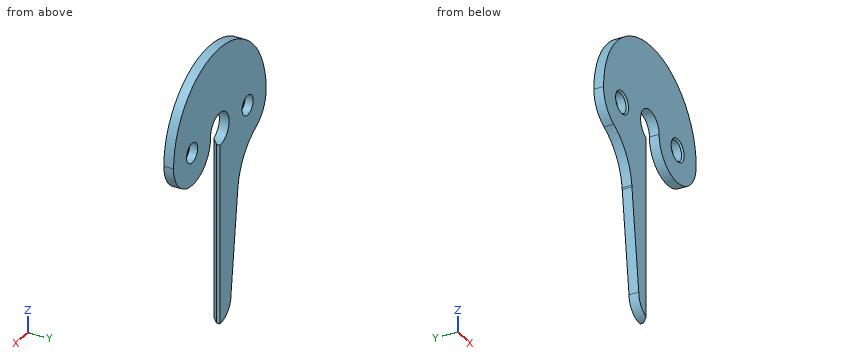
```python
from build123d import *

# Parameters (mm, degrees)
F0_R     = 3
F1_DEPTH = 3
F2_SIZE  = 2
F3_SIZE  = 0.5


with BuildPart() as f1:
    # F0 (on Front) → F1 (new body)
    with BuildSketch(Plane.XZ):
        with BuildLine():
            ThreePointArc((0, -5), (-3.535534, 3.535534), (5, 0))
            ThreePointArc((5, 0), (15, -10), (25, 0))
            ThreePointArc((25, 0), (0, 25), (-25, 0))
            ThreePointArc((-25, 0), (-23.515691, -5.242423), (-19.5034, -8.928571))
            ThreePointArc((-19.5034, -8.928571), (-12.871812, -14.665594), (-9.737763, -22.855169))
            Line((-9.737763, -22.855169), (-9.676577, -23.364999))
            Line((-9.676577, -23.364999), (-6, -54))
            ThreePointArc((-6, -54), (-4.242641, -58.242641), (0, -60))
            Line((0, -60), (0, -5))
        make_face()
        with Locations((-15, 0)):
            Circle(F0_R, mode=Mode.SUBTRACT)
        with Locations((15, 0)):
            Circle(F0_R, mode=Mode.SUBTRACT)
    extrude(amount=F1_DEPTH)

    # F2
    f2_edges = [f1.edges().sort_by_distance(p)[0] for p in [
        (0, -3, -32.5),
    ]]
    chamfer(f2_edges, length=F2_SIZE)

    # F3
    f3_edges = [f1.edges().sort_by_distance(p)[0] for p in [
        (-18, -3, 0),
        (12, -3, 0),
    ]]
    chamfer(f3_edges, length=F3_SIZE)


solid = f1.part
```
Check sheet for the modelled part. Datum: model origin and axes. Units: mm. Round coordinates to 2 decimals unless told otherwise and drop trailing zeros. Order: outer loops, then holes, each group sorted by start corner. A loop starts at its lowest first (then second) coordinate and runs counter-clockwise, first axis right, second up. Notation, with made-up numbers: (13.5, 61.5) - (62.5, 61.5) arc R30 ccw to (62.5, 90.5) - close; hole circle Ø8 at (47, 76). An arc over 180 degrees is marked (long way). Answer as CSV lines item,"result". Start each with the question number.
1) Section check A-A (x = 15). Record the cut outline in (y, z), then the cut area to 4 significant figures.
2) Section check B-B (y = -1.6). Record the cut outline in (x, z) (3 decimals), then the cut area to 3 significant figures.
3) Scan lines: probe 1 along Z at (x, y) = (15, -1.1); probe 2 along Z at (x, y) = (16, -0.05); probe 3 along X at (y, z) = (-0.2, 6). Record each from-to range of solid material in increasing order.
4) Section check D-D (x = -15). Record the cut outline in (y, z).
5) Section check C-C (z = -51). Record the cut outline in (x, y), then the cut area to 3 significant figures.
6) Depth check by flat-ended pin: pin 1 (1 mm diameter, centred on x = 4, y = -0.5, fed in from -Z); pin 2 (1 mm diameter, centred on x = 15, y = -0.5, fed in from +Z); pin 3 (0.8 mm diameter, centred on y = -0.5, z = -45.5, fed in from +X). Enter the tip coordinate at first touch or a pass-through.
Determined:
1,outline,"(-3, -10) - (0, -10) - (0, -3) - (-2.5, -3) - (-3, -3.5) - close; (-3, 3.5) - (-2.5, 3) - (0, 3) - (0, 20) - (-3, 20) - close"
1,area,"71.75 mm^2"
2,outline,"(-25, 0) arc R10 ccw to (-19.503, -8.929) arc R18 cw to (-9.738, -22.855) - (-9.677, -23.365) - (-6, -54) arc R6 ccw to (-0.6, -59.97) - (-0.6, -4.964) arc R5 cw (long way) to (5, 0) arc R10 ccw to (25, 0) arc R25 ccw to start; hole circle Ø6 at (-15, 0); hole circle Ø6 at (15, 0)"
2,area,"1,650 mm^2"
3,probe 1,"-10 to -3, 3 to 20"
3,probe 2,"-9.95 to -2.83, 2.83 to 19.21"
3,probe 3,"-24.27 to 24.27"
4,outline,"(-3, -12.15) - (0, -12.15) - (0, -3) - (-2.5, -3) - (-3, -3.5) - close; (-3, 3.5) - (-2.5, 3) - (0, 3) - (0, 20) - (-3, 20) - close"
5,outline,"(-6.36, -3) - (-2, -3) - (0, -1) - (0, 0) - (-6.36, 0) - close"
5,area,"17.1 mm^2"
6,pin 1,"z = 2.18"
6,pin 2,"z = 20.37"
6,pin 3,"x = 0"
